from build123d import *

# Parameters (mm, degrees)
SKETCH1_W           = 76.2
SKETCH1_H           = 127
BOSS_EXTRUDE1_DEPTH = 5.461
CAVITY1_START       = -38.1
CAVITY1_OUTLINE_W   = 5.461
CAVITY1_OUTLINE_H   = 25.4
CAVITY1_DEPTH       = 5.461
CAVITY1_START_2     = 32.639
CAVITY1_2_OUTLINE_W = 5.461
CAVITY1_2_OUTLINE_H = 25.4
CAVITY1_2_DEPTH     = 5.461
SKETCH2_W           = 65.278
SKETCH2_H           = 5.461
BOSS_EXTRUDE2_DEPTH = 5.461
SKETCH3_W           = 65.278
SKETCH3_H           = 5.461
BOSS_EXTRUDE3_DEPTH = 12.7


# Read off the part's stored shape, not the designer's step: Cavity1
with BuildPart() as part:
    # Sketch1 → Boss-Extrude1 (new body)
    with BuildSketch(Plane(origin=(0, 0, 0), x_dir=(1, 0, 0), z_dir=(0, 1, 0))):
        Rectangle(SKETCH1_W, SKETCH1_H)
    extrude(amount=BOSS_EXTRUDE1_DEPTH)

    # Cavity1 outline → Cavity1 (cut)
    with BuildSketch(Plane.YZ.offset(CAVITY1_START)):
        with Locations((2.7305, 25.4)):
            Rectangle(CAVITY1_OUTLINE_W, CAVITY1_OUTLINE_H)
        with Locations((2.7305, -25.4)):
            Rectangle(CAVITY1_OUTLINE_W, CAVITY1_OUTLINE_H)
    extrude(amount=CAVITY1_DEPTH, mode=Mode.SUBTRACT)

    # Cavity1 2 outline → Cavity1 2 (cut)
    with BuildSketch(Plane.YZ.offset(CAVITY1_START_2)):
        with Locations((2.7305, 25.4)):
            Rectangle(CAVITY1_2_OUTLINE_W, CAVITY1_2_OUTLINE_H)
        with Locations((2.7305, -25.4)):
            Rectangle(CAVITY1_2_OUTLINE_W, CAVITY1_2_OUTLINE_H)
    extrude(amount=CAVITY1_2_DEPTH, mode=Mode.SUBTRACT)

    # Sketch2 → Boss-Extrude2 (add)
    with BuildSketch(Plane.XY.offset(63.5)):
        with Locations((0, 2.7305)):
            Rectangle(SKETCH2_W, SKETCH2_H)
    extrude(amount=BOSS_EXTRUDE2_DEPTH)

    # Sketch3 → Boss-Extrude3 (add)
    with BuildSketch(Plane(origin=(0, 0, -63.5), x_dir=(-1, 0, 0), z_dir=(0, 0, -1))):
        with Locations((0, 2.7305)):
            Rectangle(SKETCH3_W, SKETCH3_H)
    extrude(amount=BOSS_EXTRUDE3_DEPTH)


solid = part.part
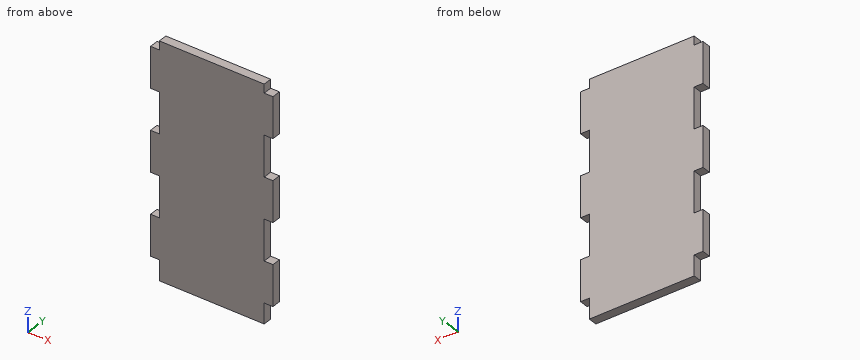
Input: part model. Units: mm. Frame: model coordinates. Coordinates: 2 decimals unless noted, no trailing zeros. Loops run counter-clockwise (first coordinate to the right, second up) from the corner with the lowest first, then second, coordinate; pieces in that order, holes last.
(1) Section A-A on y = 3.05. Return the cut outline in (x, z), then the cut area to 3 significant figures.
(2) Section B-B on z = -67. Return the cut outline in (x, y), then the cut area to 3 significant figures.
(3) First-contact query: pin 1 Ø2.5 at (x, y) = (34, 1.5) entering from +Z; pin 2 Ø2.5 at (y, z) = (2.5, 22) entering from +X; pin 3 Ø2.5 at (y, z) = (3.5, -21) entering from -X. Flat tips, straight axial feed; report the tip coordinate or a pass-through.
(4) Material intervals for probe 1 along X at (y, z) = (3.7, -15), sorted ascending.
Data:
1. outline: (-38.1, -63.5) - (-32.64, -63.5) - (-32.64, -76.2) - (32.64, -76.2) - (32.64, -63.5) - (38.1, -63.5) - (38.1, -38.1) - (32.64, -38.1) - (32.64, -12.7) - (38.1, -12.7) - (38.1, 12.7) - (32.64, 12.7) - (32.64, 38.1) - (38.1, 38.1) - (38.1, 63.5) - (32.64, 63.5) - (32.64, 68.96) - (-32.64, 68.96) - (-32.64, 63.5) - (-38.1, 63.5) - (-38.1, 38.1) - (-32.64, 38.1) - (-32.64, 12.7) - (-38.1, 12.7) - (-38.1, -12.7) - (-32.64, -12.7) - (-32.64, -38.1) - (-38.1, -38.1) - close
1. area: 10,300 mm2
2. outline: (-32.64, 0) - (32.64, 0) - (32.64, 5.46) - (-32.64, 5.46) - close
2. area: 356 mm2
3. pin 1: stops at z = 63.5
3. pin 2: stops at x = 32.64
3. pin 3: stops at x = -32.64
4. probe 1: x = -32.64 to 32.64
